from build123d import *

# Parameters (mm, degrees)
SKETCH1_W          = 2.5
SKETCH1_H          = 10
CUT_EXTRUDE1_DEPTH = 2
CHAMFER1_SIZE      = 0.2505
CHAMFER2_SIZE      = 0.9505


with BuildPart() as part:
    # Sketch1 → Revolve1 (revolve)
    with BuildSketch(Plane(origin=(0, 0, 0), x_dir=(1, 0, 0), z_dir=(0, 1, 0))):
        with Locations((1.25, 0)):
            Rectangle(SKETCH1_W, SKETCH1_H)
    revolve(axis=Axis((0, 0, -5), (0, 0, 1)))

    # Sketch2 → Cut-Extrude1 (cut)
    with BuildSketch(Plane.XY.offset(5)):
        Polygon((-0.75, -1.299038106), (0.75, -1.299038106), (1.5, 0), (0.75, 1.299038106), (-0.75, 1.299038106), (-1.5, 0), align=None)
    extrude(amount=-CUT_EXTRUDE1_DEPTH, mode=Mode.SUBTRACT)

    # Chamfer1
    chamfer1_edges = [part.edges().sort_by_distance(p)[0] for p in [
        (-2.5, 0, 5),
    ]]
    chamfer(chamfer1_edges, length=CHAMFER1_SIZE)

    # Chamfer2
    chamfer2_edges = [part.edges().sort_by_distance(p)[0] for p in [
        (-2.5, 0, -5),
    ]]
    chamfer(chamfer2_edges, length=CHAMFER2_SIZE)

    # Sketch3 → Cut-Revolve1 (revolve, cut)
    with BuildSketch(Plane(origin=(0, 0, 0), x_dir=(1, 0, 0), z_dir=(0, 1, 0))):
        Polygon((0, -3.5), (-1.5, -5), (0, -5), align=None)
    revolve(axis=Axis((0, 0, 3.5), (0, 0, -1)), mode=Mode.SUBTRACT)


solid = part.part
Design review of the part built by this model. Coordinates are the model's own, in mm. A direction names the side the tool comes from. Round coordinates to 2 decimals unless told otherwise and drop trailing zeros. Write each loop counter-clockwise with the first axis right and the second up, starting at its lowest first coordinate (ties: lowest second). Pieces come first, ordered by that corner, then holes. Notation, with made-up numbers: (74, 24) - (107, 24) arc R16 ccw to (107, 32) - close; hole circle Ø2 at (44.25, 36.5). An arc over 180 degrees is marked (long way). Use a Markdown table: item, result. Add a question column.
1. Clearance check with a flat-ended pin moving along its axis: pin 1 (0.8 mm diameter, centred on x = -0.5, z = 4, fed in from +Y). State where the tip first meets the part, or that it passes through.
2. We need section B-B (x = 0). State the section outline as (y, z) points.
3. We need section A-A (z = 3.25). State the section outline as (x, y) points.
4. Wall thickness on probe 1 along Z at (x, y) = (-0.6, -0.8); probe 2 along Y at (x, z) = (-1.1, 4.5) (3 decimals); probe 3 along X at (y, z) = (-0.7, 4): over which ranges is each line inside the solid? List them lowest first.
5. Mouldability with a two-part tool opening along Y and no side actions: class faces 3 (the face through (-0.54, -2.44, 0.29)), 4 (the face through (0, 0, 3)), 5 (the face through (0, 0, -5)) as +Y half, -Y half, draft (parallel to the pull), parting line (faces both ways), or undercut.
6. We need section C-C (z = -1.5). State the section outline as (x, y) points, then the cut area to 3 significant figures.
7. For faces 1 (the face through (0, 2, 5)), 2 (the face through (0, 1.299, 4)), list the 3-axis set-ups (+Z, -Z, +X, -X, +Y, -Y) from which the entire face can be reached by the end or side of a thin tool; tool diameter is ignored.
Output:
| question | item | result |
|---|---|---|
| 1 | pin 1 | stops at y = 2.5 |
| 2 | outline | (-2.5, -4.05) - (-1.55, -5) - (1.55, -5) - (2.5, -4.05) - (2.5, 4.75) - (2.25, 5) - (1.5, 5) - (1.3, 4.8) - (1.3, 3) - (-1.3, 3) - (-1.3, 4.8) - (-1.5, 5) - (-2.25, 5) - (-2.5, 4.75) - close |
| 3 | outline | circle Ø5 at (0, 0); hole (-1.5, 0) - (-0.75, -1.3) - (0.75, -1.3) - (1.5, 0) - (0.75, 1.3) - (-0.75, 1.3) - close |
| 4 | probe 1 | z = -5 to 3 |
| 4 | probe 2 | y = -2.245 to -0.693, 0.693 to 2.245 |
| 4 | probe 3 | x = -2.4 to -1.1, 1.1 to 2.4 |
| 5 | face 3 | parting line |
| 5 | face 4 | undercut |
| 5 | face 5 | draft |
| 6 | outline | circle Ø5 at (0, 0) |
| 6 | area | 19.6 mm2 |
| 7 | face 1 | +Z, +X, -X, +Y, -Y |
| 7 | face 2 | +Z |
